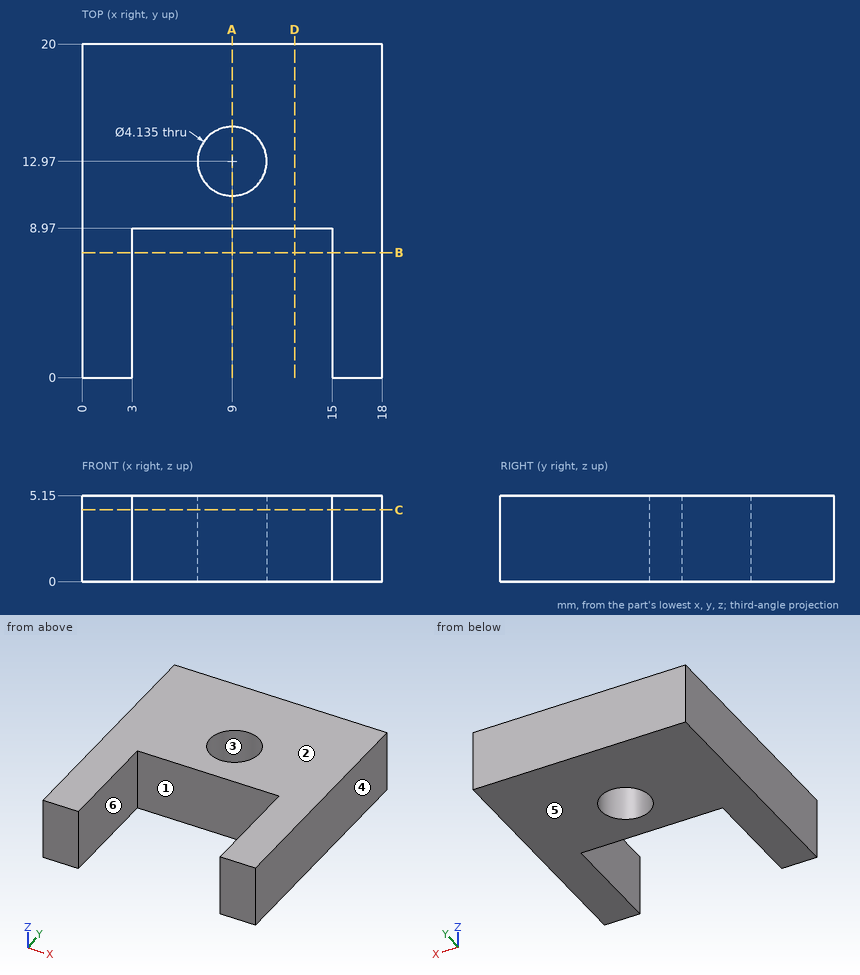
Here's the drawing with two shaded views (mm, measured from the low corner). I have some questions. A direction names the side the tool comes from. Round coordinates to 2 decimals unless told otherwise and drop trailing zeros. Loops run counter-clockwise (first coordinate to the right, second up) from the corner with the lowest first, then second, coordinate; pieces in that order, holes last. Notation, with made-up numbers: M -23,88.5 L -3,88.5 A9 ccw -3,103.5 Z; hole C 48,44 d9. An arc over 180 degrees is marked long. Put each result on its own line as item: value.
Q1. Thinking about a two-plate mould opening in X: for the marked faces 1, 2, 3 and 4, which applies, released by +X, released by -X, zero draft, split by the parting line, or undercut?
Check result:
face 1: undercut
face 2: zero draft
face 3: undercut
face 4: released by +X
Q2. Imagine slicing it at D-D (x = 12.75). Write out the boundary of the cut face in (y, z), then the cut area to 3 significant figures.
Check result:
outline: M 8.97,0 L 20,0 L 20,5.15 L 8.97,5.15 Z
area: 56.8 mm2
Q3. Imagine slicing it at A-A (x = 9). Write out the boundary of the cut face in (y, z).
Check result:
outline: M 8.97,0 L 10.9,0 L 10.9,5.15 L 8.97,5.15 Z; M 15.04,0 L 20,0 L 20,5.15 L 15.04,5.15 Z
Q4. For pin 1 (2 mm diameter, centred on x = 6.5, z = 1.5, fed in from -Y), with a flat end and sliding along its axis, tell me the tip position at first contact or that it passes through.
Check result:
pin 1: y = 8.97
Q5. Imagine slicing it at B-B (y = 7.5). Write out the boundary of the cut face in (x, z).
Check result:
outline: M 0,0 L 3,0 L 3,5.15 L 0,5.15 Z; M 15,0 L 18,0 L 18,5.15 L 15,5.15 Z
Q6. I need wall thicknesses on probe 1 along X at (y, z) = (8.5, 2.2); probe 2 along Y at (x, z) = (9, 2.8); probe 3 along Y at (x, z) = (4.75, 2.9). Which ranges of each line are inside material? Lowest first, please.
Check result:
probe 1: 0 to 3, 15 to 18
probe 2: 8.97 to 10.9, 15.04 to 20
probe 3: 8.97 to 20
Q7. Imagine slicing it at C-C (z = 4.3). Write out the boundary of the cut face in (x, y) (1 decimal), then the cut area to 3 significant figures.
Check result:
outline: M 0,0 L 3,0 L 3,9 L 15,9 L 15,0 L 18,0 L 18,20 L 0,20 Z; hole C 9,13 d4.1
area: 239 mm2
Q8. On a 3-axis mill with a long thin cutter (end or side, diameter ignored), from which of +Z, -Z, +X, -X, +Y, -Y can I reach the whole of each face in a straight line? I mean the marked faces 5 and 6. Say none if no direction works.
Check result:
face 5: -Z, +X, -X, +Y, -Y
face 6: +Z, -Z, -Y
